from build123d import *

# Parameters (mm, degrees)
SKETCH1_W               = 75
SKETCH1_H               = 65
BOSS_EXTRUDE1_DEPTH     = 55
SKETCH2_W               = 28
SKETCH2_H               = 44
BOSS_EXTRUDE2_DEPTH     = 18
CHAMFER1_SIZE           = 12
CUT_EXTRUDE1_DEPTH      = 77.154844523
CUT_EXTRUDE1_DEPTH_BACK = 77.154844523
SKETCH3_R               = 1


with BuildPart() as part:
    # Sketch1 → Boss-Extrude1 (new body)
    with BuildSketch(Plane.YZ):
        with Locations((5.396678967, -3.201107011)):
            Rectangle(SKETCH1_W, SKETCH1_H)
    extrude(amount=BOSS_EXTRUDE1_DEPTH)

    # Sketch2 → Boss-Extrude2 (add)
    with BuildSketch(Plane.XY.offset(29.298892989)):
        with Locations((27.5, 5.396678967)):
            Rectangle(SKETCH2_W, SKETCH2_H)
    extrude(amount=BOSS_EXTRUDE2_DEPTH)

    # Chamfer1
    chamfer1_edges = [part.edges().sort_by_distance(p)[0] for p in [
        (55, 5.396678967, 29.298892989),
        (0, 5.396678967, 29.298892989),
        (0, 5.396678967, -35.701107011),
        (27.5, -32.103321033, 29.298892989),
        (27.5, 42.896678967, 29.298892989),
        (27.5, 42.896678967, -35.701107011),
        (27.5, -32.103321033, -35.701107011),
        (55, 5.396678967, -35.701107011),
    ]]
    chamfer(chamfer1_edges, length=CHAMFER1_SIZE)

    # Sketch3 → Cut-Extrude1 (cut, two sides: drawn at the far end of the back side and taken through both)
    with BuildSketch(Plane.YZ.offset(41.5).offset(-CUT_EXTRUDE1_DEPTH_BACK)):
        with Locations((5.396678967, 38.298892989)):
            Circle(SKETCH3_R)
    extrude(amount=CUT_EXTRUDE1_DEPTH + CUT_EXTRUDE1_DEPTH_BACK, mode=Mode.SUBTRACT)


solid = part.part
Design review of the part built by this model. Coordinates are the model's own, in mm. A direction names the side the tool comes from. Coordinates: 2 decimals unless noted, no trailing zeros. Loops run counter-clockwise (first coordinate to the right, second up) from the corner with the lowest first, then second, coordinate; pieces in that order, holes last. Notation, with made-up numbers: (75, 82.25) -> (99, 82.25) arc R4 cw to (99, 88.25) -> close; hole circle Ø4 at (55, 30.5). An arc over 180 degrees is marked (long way). Use a Markdown table: item, result. Add a question column.
Item 1: We need section A-A, the plane y = 29. Write out the cut boundary in (x, z), and give its area (3 significant figures).
Item 2: We need section B-B, the plane x = 51.5. Write out the cut boundary in (y, z), and give its area (3 significant figures).
Item 3: The part is to be moulded in two halves that separate along Y. For faces 4 (the flat face through (27, 42.897, -3)), 5 (the cylindrical face through (27.304, 5.18, 37.323)), 6 (the flat face through (27, -32.103, -3)), 7 (the flat face through (55, 5, -3)), say which applies: +Y half, -Y half, draft (parallel to the pull), parting line (faces both ways), or undercut.
Item 4: Wall thickness on L1, parallel to Y at x = 19, z = 42; L2, parallel to Z at x = 18, y = -18.5; L3, parallel to Z at x = 27, y = 31: over which ranges is each line inside the solid? List them lowest first. Write a range as from..to.
Item 5: We need section C-C, the plane x = 29. Write out the cut boundary in (y, z).
Item 6: We need section D-D, the plane y = -7.5. Write out the cut boundary in (x, z), and give its area (3 significant figures).
Item 7: Machinability: for faces 1 (the flat face through (41.5, 5, 40)), 2 (the flat face through (13.5, 5, 40)), 3 (the flat face through (27, -16.603, 38)), which of the approach directions +Z, -Z, +X, -X, +Y, -Y give a long, thin tool a straight path to every point of the face, cutting with its end or side? Answer none if there is none.
Item 8: Clearance check with flat-ended pins moving along their axes: P1, Ø2, axis at y = 33.5, z = -25.5, coming from the -X side; P2, Ø2.5, axis at y = 5.4, z = 38.3, coming from the -X side; P3, Ø5, axis at x = 15, z = 30, coming from the -Y side. State where each tip first meets the part, or that it passes through.
Numbers:
| question | item | result |
|---|---|---|
| 1 | outline | (0, -23.7) -> (12, -35.7) -> (43, -35.7) -> (55, -23.7) -> (55, 17.3) -> (43, 29.3) -> (12, 29.3) -> (0, 17.3) -> close |
| 1 | area | 3,290 mm^2 |
| 2 | outline | (-32.1, -23.7) -> (-28.6, -27.2) -> (39.4, -27.2) -> (42.9, -23.7) -> (42.9, 17.3) -> (39.4, 20.8) -> (-28.6, 20.8) -> (-32.1, 17.3) -> close |
| 2 | area | 3,580 mm^2 |
| 3 | face 4 | +Y half |
| 3 | face 5 | undercut |
| 3 | face 6 | -Y half |
| 3 | face 7 | draft |
| 4 | L1 | y = -16.6..27.4 |
| 4 | L2 | z = -35.7..29.3 |
| 4 | L3 | z = -35.6..29.2 |
| 5 | outline | (-32.1, -23.7) -> (-20.1, -35.7) -> (30.9, -35.7) -> (42.9, -23.7) -> (42.9, 17.3) -> (30.9, 29.3) -> (27.4, 29.3) -> (27.4, 47.3) -> (-16.6, 47.3) -> (-16.6, 29.3) -> (-20.1, 29.3) -> (-32.1, 17.3) -> close; hole circle Ø2 at (5.4, 38.3) |
| 6 | outline | (0, -23.7) -> (12, -35.7) -> (43, -35.7) -> (55, -23.7) -> (55, 17.3) -> (43, 29.3) -> (41.5, 29.3) -> (41.5, 47.3) -> (13.5, 47.3) -> (13.5, 29.3) -> (12, 29.3) -> (0, 17.3) -> close |
| 6 | area | 3,790 mm^2 |
| 7 | face 1 | +Z, +X, +Y, -Y |
| 7 | face 2 | +Z, -X, +Y, -Y |
| 7 | face 3 | +Z, +X, -X, -Y |
| 8 | P1 | stops at x = 0.8 |
| 8 | P2 | stops at x = 13.5 |
| 8 | P3 | stops at y = -21.9 |
